Source: three-view drawing plus pictorial views. Frame: mm from the lowest corner of the part. A direction names the side the tool comes from. Coordinates: 2 decimals unless noted, no trailing zeros. Write each loop counter-clockwise with the first axis right and the second up, starting at its lowest first coordinate (ties: lowest second). Pieces come first, ordered by that corner, then holes. Notation, with made-up numbers: (48.25, -23.5) - (74.25, -23.5) arc R25 ccw to (74.25, -10.5) - close; hole circle Ø2 at (-35, -24.5). An arc over 180 degrees is marked (long way). One line per item, written item: value.
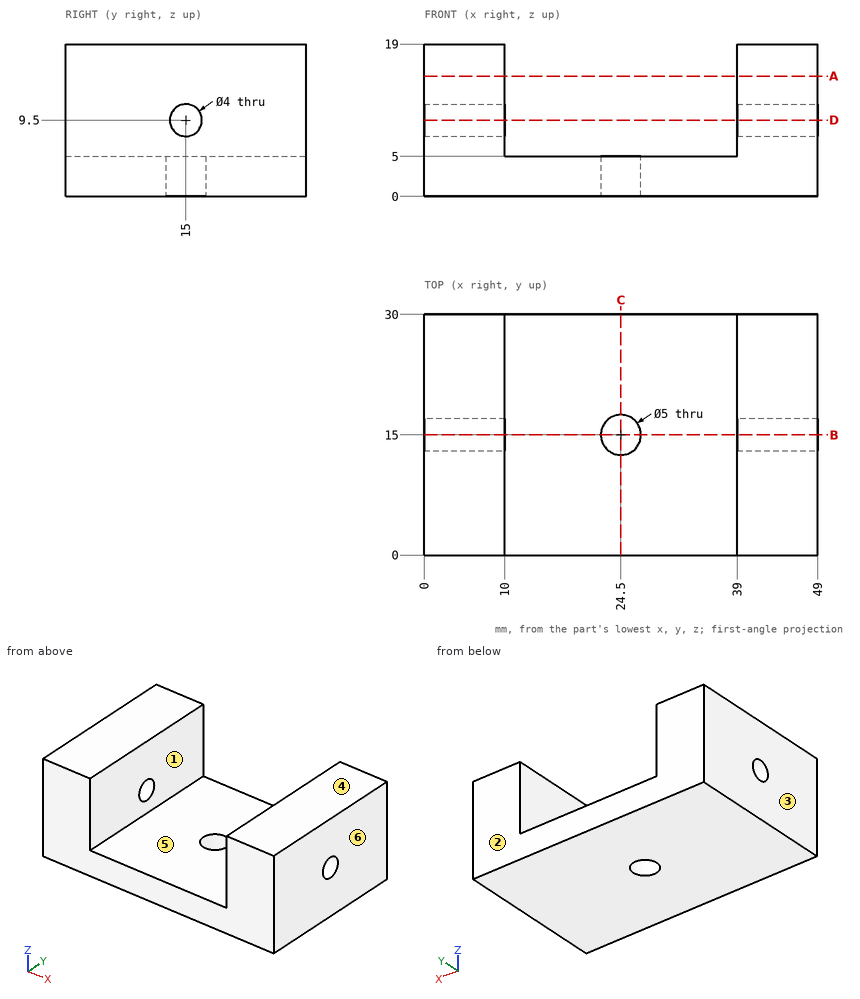
1) Draft query along X for the marked faces 3, 4, 5 and 6. Return one class per face: released by +X, released by -X, zero draft, split by the parting line, or undercut.
Values found:
face 3: released by -X
face 4: zero draft
face 5: undercut
face 6: released by +X
2) Section query A-A on z = 15. Output: boundary loops of the cut face in (x, y).
Values found:
outline: (0, 0) - (10, 0) - (10, 30) - (0, 30) - close; (39, 0) - (49, 0) - (49, 30) - (39, 30) - close
3) Material intervals for line 1 (X direction, y = 28, z = 10); line 2 (Z direction, x = 46, y = 15); line 3 (Z direction, x = 33, y = 12.25), sorted ascending.
Values found:
line 1: 0 to 10, 39 to 49
line 2: 0 to 7.5, 11.5 to 19
line 3: 0 to 5
4) Contact query for flat-ended pins moving along their axis: P1, Ø4, axis at x = 15.5, y = 17.5, coming from the +Z side; P2, Ø3, axis at y = 15, z = 9.5, coming from the +X side. Output: stop coordinate, or through.
Values found:
P1: z = 5
P2: through
5) Reachability of the marked faces 1 and 2 from +Z, -Z, +X, -X, +Y, -Y: full face, straight path, thin tool, end or side. Return the list, or none.
Values found:
face 1: +Z, +Y, -Y
face 2: +Z, -Z, +X, -X, +Y
6) Section query B-B on y = 15. Output: boundary loops of the cut face in (x, z), then the cut area to 3 significant figures.
Values found:
outline: (0, 0) - (22, 0) - (22, 5) - (10, 5) - (10, 7.5) - (0, 7.5) - close; (0, 11.5) - (10, 11.5) - (10, 19) - (0, 19) - close; (27, 0) - (49, 0) - (49, 7.5) - (39, 7.5) - (39, 5) - (27, 5) - close; (39, 11.5) - (49, 11.5) - (49, 19) - (39, 19) - close
area: 420 mm2
7) Section query D-D on z = 9.5. Output: boundary loops of the cut face in (x, y), then the cut area to 3 significant figures.
Values found:
outline: (0, 0) - (10, 0) - (10, 13) - (0, 13) - close; (0, 17) - (10, 17) - (10, 30) - (0, 30) - close; (39, 0) - (49, 0) - (49, 13) - (39, 13) - close; (39, 17) - (49, 17) - (49, 30) - (39, 30) - close
area: 520 mm2
8) Section query C-C on x = 24.5. Output: boundary loops of the cut face in (y, z), then the cut area to 3 significant figures.
Values found:
outline: (0, 0) - (12.5, 0) - (12.5, 5) - (0, 5) - close; (17.5, 0) - (30, 0) - (30, 5) - (17.5, 5) - close
area: 125 mm2
